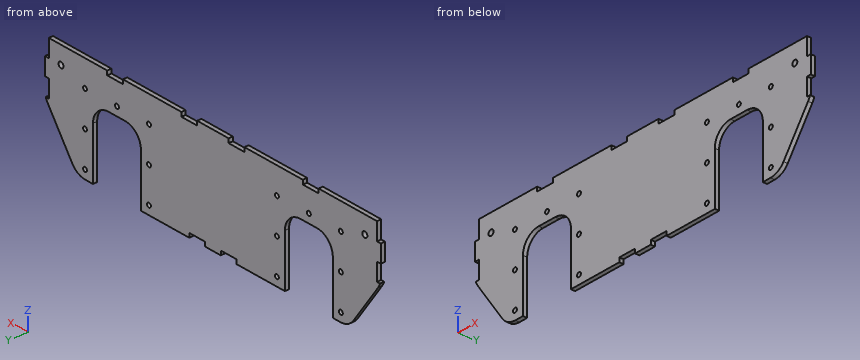
```python
from build123d import *

# Parameters (mm, degrees)
F1_DEPTH = 6
F2_W     = 6
F2_H     = 25
F2_W_2   = 25
F2_H_2   = 6
F3_DEPTH = 25
F5_D     = 6.2
F6_D     = 8


with BuildPart() as f1:
    # F0 (on Front) → F1 (new body)
    with BuildSketch(Plane.XZ):
        with BuildLine():
            Line((224.8010802506, 50.9528913677), (-308.5989197494, 50.9528913677))
            Line((-308.5989197494, 50.9528913677), (-308.5989197494, -16.3773312117))
            ThreePointArc((-308.5989197494, -16.3773312117), (-307.4994411864, -23.709798398), (-304.2977137462, -30.3973143456))
            Line((-304.2977137462, -30.3973143456), (-265.2360511733, -88.0670917662))
            ThreePointArc((-265.2360511733, -88.0670917662), (-256.2526406882, -96.1321666846), (-244.5372571765, -99.0471086323))
            Line((-244.5372571765, -99.0471086323), (-232.3989197494, -99.0471086323))
            Line((-232.3989197494, -99.0471086323), (-232.3989197494, -24.0471086323))
            ThreePointArc((-232.3989197494, -24.0471086323), (-225.076589279, -6.3694391026), (-207.3989197494, 0.9528913677))
            Line((-207.3989197494, 0.9528913677), (-181.1989197494, 0.9528913677))
            ThreePointArc((-181.1989197494, 0.9528913677), (-163.5212502197, -6.3694391026), (-156.1989197494, -24.0471086323))
            Line((-156.1989197494, -24.0471086323), (-156.1989197494, -99.0471086323))
            Line((-156.1989197494, -99.0471086323), (72.4010802506, -99.0471086323))
            Line((72.4010802506, -99.0471086323), (72.4010802506, -24.0471086323))
            ThreePointArc((72.4010802506, -24.0471086323), (79.723410721, -6.3694391026), (97.4010802506, 0.9528913677))
            Line((97.4010802506, 0.9528913677), (123.6010802506, 0.9528913677))
            ThreePointArc((123.6010802506, 0.9528913677), (141.2787497803, -6.3694391026), (148.6010802506, -24.0471086323))
            Line((148.6010802506, -24.0471086323), (148.6010802506, -99.0471086323))
            Line((148.6010802506, -99.0471086323), (160.7394176777, -99.0471086323))
            ThreePointArc((160.7394176777, -99.0471086323), (172.4548011894, -96.1321666846), (181.4382116746, -88.0670917662))
            Line((181.4382116746, -88.0670917662), (220.4998742475, -30.3973143456))
            ThreePointArc((220.4998742475, -30.3973143456), (223.7016016877, -23.709798398), (224.8010802506, -16.3773312117))
            Line((224.8010802506, -16.3773312117), (224.8010802506, 50.9528913677))
        make_face()
    extrude(amount=F1_DEPTH)

    # F2 (on face) → F3 (cut)
    with BuildSketch(Plane.XZ.offset(6)):
        with Locations((-305.5989197494, 38.4528913677)):
            Rectangle(F2_W, F2_H)
        with Locations((-305.5989197494, -11.5471086323)):
            Rectangle(F2_W, F2_H)
        with Locations((221.8010802506, 38.4528913677)):
            Rectangle(F2_W, F2_H)
        with Locations((221.8010802506, -11.5471086323)):
            Rectangle(F2_W, F2_H)
        with Locations((-66.8989197494, -96.0471086323)):
            Rectangle(F2_W_2, F2_H_2)
        with Locations((-16.8989197494, -96.0471086323)):
            Rectangle(F2_W_2, F2_H_2)
        with Locations((-79.3989197494, 47.9528913677)):
            Rectangle(F2_W_2, F2_H_2)
        with Locations((-4.3989197494, 47.9528913677)):
            Rectangle(F2_W_2, F2_H_2)
        with Locations((-197.2489197494, 47.9528913677)):
            Rectangle(F2_W_2, F2_H_2)
        with Locations((113.4510802506, 47.9528913677)):
            Rectangle(F2_W_2, F2_H_2)
    extrude(amount=-F3_DEPTH, mode=Mode.SUBTRACT)

    # F5 (through all)
    with Locations(Plane.XZ.offset(6)):
        with Locations((-245.0989197494, -86.5471086323), (-245.0989197494, -36.5471086323), (-245.0989197494, 13.4528913677), (-194.2989197494, 13.4528913677), (-143.4989197494, 13.4528913677), (-143.4989197494, -36.5471086323), (-143.4989197494, -86.5471086323), (59.7010802506, -86.5471086323), (59.7010802506, -36.5471086323), (59.7010802506, 13.4528913677), (110.5010802506, 13.4528913677), (161.3010802506, 13.4528913677), (161.3010802506, -36.5471086323), (161.3010802506, -86.5471086323)):
            Hole(F5_D / 2)

    # F6 (through all)
    with Locations(Plane.XZ.offset(6)):
        with Locations((-283.1989197494, 25.9528913677), (199.4010802506, 25.9528913677)):
            Hole(F6_D / 2)


solid = f1.part
```
Part model, mm, in its own coordinate system. Coordinates: 2 decimals unless noted, no trailing zeros. Order: outer loops, then holes, each group sorted by start corner. A loop starts at its lowest first (then second) coordinate and runs counter-clockwise, first axis right, second up. Notation, with made-up numbers: (-28, 45) - (10, 45) arc R19 cw to (10, 66) - close; hole circle Ø6 at (21.5, 2.5). An arc over 180 degrees is marked (long way). Return JSON: item names as keys, results as strings. Group by question number.
Item 1: Cut at C-C (y = -3.2). State how many separate pieces and enclosed holes the cut face has, plus the area to 3 significant figures.
Item 2: Cut at A-A (z = -12). List the corners of the cut face in (x, y).
Item 3: Cut at B-B (z = -60). List the corners of the cut face in (x, y), plus the area to 3 significant figures.
Item 4: Pin check, flat tips, straight feed: pin 1 (3 mm diameter, centred on y = -3.5, z = -35, fed in from -X); pin 2 (3 mm diameter, centred on y = -3.5, z = -77.5, fed in from +X); pin 3 (3 mm diameter, centred on y = -4, z = 39.5, fed in from -X). Stop position of each tip, or through.
Item 5: Drill centre lines: probe 1 along X at (y, z) = (-2.75, -80); probe 2 along X at (y, z) = (-1.9, -31); probe 3 along X at (y, z) = (-1.15, 44). Where is each one in solid material? Low to high. Write a range as from..to.
Check values:
{
 "1": {"separate pieces": "1", "enclosed holes": "16", "area": "59,400 mm2"},
 "2": {"outline": "(-302.6, -6) - (-229.3, -6) - (-229.3, 0) - (-302.6, 0) - close; (-159.29, -6) - (75.5, -6) - (75.5, 0) - (-159.29, 0) - close; (145.51, -6) - (218.8, -6) - (218.8, 0) - (145.51, 0) - close"},
 "3": {"outline": "(-284.25, -6) - (-232.4, -6) - (-232.4, 0) - (-284.25, 0) - close; (-156.2, -6) - (72.4, -6) - (72.4, 0) - (-156.2, 0) - close; (148.6, -6) - (200.45, -6) - (200.45, 0) - (148.6, 0) - close", "area": "1,990 mm2"},
 "4": {"pin 1": "stops at x = -302.2", "pin 2": "stops at x = 189.61", "pin 3": "stops at x = -302.6"},
 "5": {"probe 1": "x = -270.7..-232.4, -156.2..72.4, 148.6..186.9", "probe 2": "x = -303.89..-232.4, -156.2..72.4, 148.6..220.09", "probe 3": "x = -302.6..218.8"}
}
